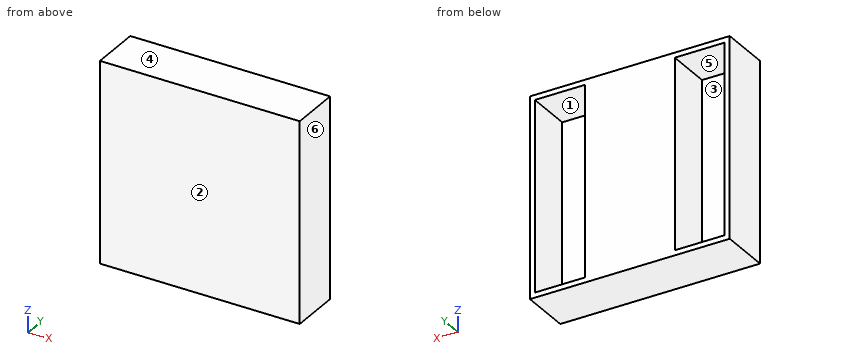
Autodesk Inventor part; units mm, degrees
ref_plane "YZ Plane" through (0, 0, 0) normal (1, 0, 0) x (0, 1, 0)
ref_plane "XZ Plane" through (0, 0, 0) normal (0, 1, 0) x (-1, 0, 0)
ref_plane "XY Plane" through (0, 0, 0) normal (0, 0, 1) x (1, 0, 0)
sketch "Sketch1" plane through (0, 0, 0) normal (0, 1, 0) x (-1, 0, 0)
  line L0 (0, 0) -> (200, 0)
  line L1 (200, 0) -> (200, -200)
  line L2 (200, -200) -> (0, -200)
  line L3 (0, -200) -> (0, 0)
  dimension "d0" = 200
  dimension "d1" = 200
extrude "Extrusion1" add sketch "Sketch1" along normal blind 50
sketch "Sketch2" plane through (0, 50, 0) normal (0, 1, 0) x (1, 0, 0)
  line L0 (-5, 5) -> (-5, 195)
  line L1 (0, 200) -> (-200, 200)
  line L2 (-5, 195) -> (-55, 195)
  line L3 (-55, 195) -> (-55, 5)
  line L4 (-55, 5) -> (-5, 5)
  line L5 (-200, 200) -> (-200, 0)
  line L6 (-195, 195) -> (-145, 195)
  line L7 (-145, 195) -> (-145, 5)
  line L8 (-145, 5) -> (-195, 5)
  line L9 (-195, 5) -> (-195, 195)
  point P0 (0, 0)
  dimension "d4" = 190
  dimension "d5" = 50
  dimension "d16" = 50
  dimension "d17" = 190
  dimension "d20" = 5
extrude "Extrusion2" cut sketch "Sketch2" against normal blind 45 contours L4 L3 L2 L0
extrude "Extrusión4" cut sketch "Sketch2" against normal blind 45 contours L6 L7 L8 L9
properties part number "Box"
CAD build for the part. Positions are in the model's coordinates, mm. Face numbers are marked on the shaded views. A direction names the side the tool comes from. Round coordinates to 2 decimals unless told otherwise and drop trailing zeros. Write each loop counter-clockwise with the first axis right and the second up, starting at its lowest first coordinate (ties: lowest second). Pieces come first, ordered by that corner, then holes. Notation, with made-up numbers: (-5, 24) - (38, 24) arc R5 cw to (38, 31) - close; hole circle Ø10 at (-25.5, 81.25). An arc over 180 degrees is marked (long way). Return JSON: item names as keys, results as strings. Group by question number.
Item 1: Band-saw the part on B-B on z = -79. List the corners of the cut face in (x, y).
Item 2: Probe probe 1 along X at (y, z) = (8.5, -20); probe 2 along Z at (x, y) = (-169, 27); probe 3 along Y at (x, z) = (-156, -23). List the from-to ranges inside material, lowest first.
Item 3: Band-saw the part on A-A on y = 40.5. List the corners of the cut face in (x, z), plus the area to 3 significant figures.
Item 4: Mould opens along Z. For the marked faces 3, 4, 5 and 6 say: +Z half, -Z half, draft (parallel to the pull), parting line (faces both ways), or undercut.
Item 5: 3-axis set-ups, long thin cutter, end or side, ignore diameter. For the marked faces 1 and 2: which of +Z, -Z, +X, -X, +Y, -Y reach the whole face in a straight line?
Item 6: Flat gauge pin, fed straight in: pin 1 Ø1 at (x, z) = (-32.5, -59.5) entering from -Y. Where does the tip first touch, or does it go through?
Resolved:
{
 "1": {"outline": "(-200, 0) - (0, 0) - (0, 50) - (-5, 50) - (-5, 5) - (-55, 5) - (-55, 50) - (-145, 50) - (-145, 5) - (-195, 5) - (-195, 50) - (-200, 50) - close"},
 "2": {"probe 1": "x = -200 to -195, -145 to -55, -5 to 0", "probe 2": "z = -200 to -195, -5 to 0", "probe 3": "y = 0 to 5"},
 "3": {"outline": "(-200, -200) - (0, -200) - (0, 0) - (-200, 0) - close; hole (-195, -195) - (-145, -195) - (-145, -5) - (-195, -5) - close; hole (-55, -195) - (-5, -195) - (-5, -5) - (-55, -5) - close", "area": "21,000 mm²"},
 "4": {"face 3": "undercut", "face 4": "+Z half", "face 5": "undercut", "face 6": "draft"},
 "5": {"face 1": "+Y", "face 2": "+Z, -Z, +X, -X, -Y"},
 "6": {"pin 1": "stops at y = 0"}
}
